```python
from build123d import *

# Parameters (mm, degrees)
SKETCH1_W           = 230
SKETCH1_H           = 230
BOSS_EXTRUDE1_DEPTH = 20
SKETCH2_W           = 20
SKETCH2_H           = 10
SKETCH2_H_2         = 90
CUT_EXTRUDE1_DEPTH  = 20
SKETCH3_R           = 5
CUT_EXTRUDE2_DEPTH  = 210
FILLET1_R           = 5
FILLET2_R           = 5


with BuildPart() as part:
    # Sketch1 → Boss-Extrude1 (new body)
    with BuildSketch(Plane(origin=(0, 0, 0), x_dir=(0, 0, -1), z_dir=(1, 0, 0))):
        Rectangle(SKETCH1_W, SKETCH1_H)
    extrude(amount=BOSS_EXTRUDE1_DEPTH)

    # Sketch2 → Cut-Extrude1 (cut)
    with BuildSketch(Plane.XY.offset(115)):
        with Locations((10, 110)):
            Rectangle(SKETCH2_W, SKETCH2_H)
        with Locations((10, 50)):
            Rectangle(SKETCH2_W, SKETCH2_H_2)
        with Locations((10, -50)):
            Rectangle(SKETCH2_W, SKETCH2_H_2)
        with Locations((10, -110)):
            Rectangle(SKETCH2_W, SKETCH2_H)
    cut_extrude1 = extrude(amount=-CUT_EXTRUDE1_DEPTH, mode=Mode.SUBTRACT)

    # Sketch3 → Cut-Extrude2 (cut)
    with BuildSketch(Plane(origin=(0, 105, 0), x_dir=(1, 0, 0), z_dir=(0, 1, 0))):
        with Locations((10, -105)):
            Circle(SKETCH3_R)
    cut_extrude2 = extrude(amount=-CUT_EXTRUDE2_DEPTH, mode=Mode.SUBTRACT)

    # Fillet1
    fillet1_edges = [part.edges().sort_by_distance(p)[0] for p in [
        (0, 100, 115),
        (0, 0, 115),
        (0, -100, 115),
        (20, 100, 115),
        (20, 0, 115),
        (20, -100, 115),
    ]]
    fillet(fillet1_edges, radius=FILLET1_R)

    # Mirror5: Cut-Extrude1, Cut-Extrude2 across plane
    add(cut_extrude1.mirror(Plane.XY), mode=Mode.SUBTRACT)
    add(cut_extrude2.mirror(Plane.XY), mode=Mode.SUBTRACT)

    # Fillet2
    fillet2_edges = [part.edges().sort_by_distance(p)[0] for p in [
        (0, -100, -115),
        (0, 0, -115),
        (0, 100, -115),
        (20, -100, -115),
        (20, 0, -115),
        (20, 100, -115),
    ]]
    fillet(fillet2_edges, radius=FILLET2_R)


solid = part.part
```
Design review of the part built by this model. Coordinates are the model's own, in mm. A direction names the side the tool comes from. Round coordinates to 2 decimals unless told otherwise and drop trailing zeros. Write each loop counter-clockwise with the first axis right and the second up, starting at its lowest first coordinate (ties: lowest second). Pieces come first, ordered by that corner, then holes.
Item 1: We need section B-B on y = -99. Write out the cut boundary in (x, z), and give its area (3 significant figures).
Item 2: Clearance check with flat-ended pins moving along their axes: pin 1 Ø10 at (x, z) = (10.5, 105) entering from +Y; pin 2 Ø6 at (x, y) = (12.5, 24) entering from -Z; pin 3 Ø6 at (x, z) = (14, 100.5) entering from -Y. State where each tip first meets the part, or that it passes through.
Item 3: For probe 1 along Y at (x, z) = (6, 99); probe 2 along X at (y, z) = (102, -105); probe 3 along Z at (x, y) = (10, 99.5), list the stretches that pass through material, from the lowest coordinate up.
Item 4: We need section C-C on x = 10. State how many separate pieces and enclosed holes the cut face has, and give its area (3 significant figures).
Item 5: For faces 1 (the flat face through (10, -49, 95)), 2 (the flat face through (10, -49, -95)), 3 (the flat face through (10, -110, -95)), list the 3-axis set-ups (+Z, -Z, +X, -X, +Y, -Y) from which the entire face can be reached by the end or side of a thin tool; tool diameter is ignored.
Item 6: We need section A-A on z = -105. Write out the cut boundary in (x, y).
Item 7: The part is to be moulded in two halves that separate along Y. For faces 4 (the flat face through (10, 115, 1)), 5 (the flat face through (5, -95, -103)), 6 (the flat face through (10, 0, 115)), say which applies: +Y half, -Y half, draft (parallel to the pull), parting line (faces both ways), or undercut.
Returned:
1. outline: (0, -110) arc R5 ccw to (5, -115) - (15, -115) arc R5 ccw to (20, -110) - (20, 110) arc R5 ccw to (15, 115) - (5, 115) arc R5 ccw to (0, 110) - close; hole circle Ø10 at (10, -105); hole circle Ø10 at (10, 105)
1. area: 4,420 mm2
2. pin 1: stops at y = 105
2. pin 2: stops at z = -95
2. pin 3: stops at y = -105
3. probe 1: y = -105 to -95, -5 to 5, 95 to 105
3. probe 2: x = 0 to 5, 15 to 20
3. probe 3: z = -115 to -110, -100 to 100, 110 to 115
4. separate pieces: 7
4. enclosed holes: 0
4. area: 44,300 mm2
5. face 1: +Z, +X, -X
5. face 2: -Z, +X, -X
5. face 3: -Z, +X, -X, -Y
6. outline: (0, -105) - (5, -105) - (5, -95) - (0, -95) - close; (0, -5) - (5, -5) - (5, 5) - (0, 5) - close; (0, 95) - (5, 95) - (5, 105) - (0, 105) - close; (15, -105) - (20, -105) - (20, -95) - (15, -95) - close; (15, -5) - (20, -5) - (20, 5) - (15, 5) - close; (15, 95) - (20, 95) - (20, 105) - (15, 105) - close
7. face 4: +Y half
7. face 5: undercut
7. face 6: draft
